from build123d import *

# Parameters (mm, degrees)
SKETCH2_W           = 180
SKETCH2_H           = 300
BOSS_EXTRUDE1_DEPTH = 3
SKETCH3_W           = 8.2
SKETCH3_H           = 260
CUT_EXTRUDE1_DEPTH  = 175.954279742
SKETCH4_R           = 2.5
CUT_EXTRUDE2_DEPTH  = 175.954279742


with BuildPart() as part:
    # Sketch2 → Boss-Extrude1 (new body)
    with BuildSketch(Plane(origin=(0, 0, 0), x_dir=(1, 0, 0), z_dir=(0, 1, 0))):
        Rectangle(SKETCH2_W, SKETCH2_H)
    extrude(amount=BOSS_EXTRUDE1_DEPTH)

    # Sketch3 → Cut-Extrude1 (cut, through all)
    with BuildSketch(Plane(origin=(0, 3, 0), x_dir=(1, 0, 0), z_dir=(0, 1, 0))):
        with Locations((-67.5, 0)):
            Rectangle(SKETCH3_W, SKETCH3_H)
        with Locations((-22.5, 0)):
            Rectangle(SKETCH3_W, SKETCH3_H)
        with Locations((22.5, 0)):
            Rectangle(SKETCH3_W, SKETCH3_H)
        with Locations((67.5, 0)):
            Rectangle(SKETCH3_W, SKETCH3_H)
    extrude(amount=-CUT_EXTRUDE1_DEPTH, mode=Mode.SUBTRACT)

    # Sketch4 → Cut-Extrude2 (cut, through all)
    with BuildSketch(Plane(origin=(0, 3, 0), x_dir=(1, 0, 0), z_dir=(0, 1, 0))):
        with Locations(Location((67.5, -140, 0), (0, 0, 270))):
            Circle(SKETCH4_R)
        with Locations(Location((-67.5, -140, 0), (0, 0, 90))):
            Circle(SKETCH4_R)
        with Locations(Location((67.5, 140, 0), (0, 0, 90))):
            Circle(SKETCH4_R)
        with Locations(Location((-67.5, 140, 0), (0, 0, 270))):
            Circle(SKETCH4_R)
        with Locations(Location((-22.5, -140, 0), (0, 0, 270))):
            Circle(SKETCH4_R)
        with Locations(Location((22.5, -140, 0), (0, 0, 90))):
            Circle(SKETCH4_R)
        with Locations(Location((22.5, 140, 0), (0, 0, 270))):
            Circle(SKETCH4_R)
        with Locations(Location((-22.5, 140, 0), (0, 0, 90))):
            Circle(SKETCH4_R)
    extrude(amount=-CUT_EXTRUDE2_DEPTH, mode=Mode.SUBTRACT)


solid = part.part
Could you check a few things on this model? Use its own coordinates, in mm. Give positions to 0.01 mm unless a question says otherwise; leave off trailing zeros. Order: outer loops, then holes, each group sorted by start corner. A loop starts at its lowest first (then second) coordinate and runs counter-clockwise, first axis right, second up.
1. I need wall thicknesses on L1, parallel to X at y = 1.95, z = 140; L2, parallel to X at y = 1.85, z = -117. Which ranges of each line are inside material? Lowest first, please.
2. Suppose I cut it at A-A (y = 0.75). Give the number of separate pieces and of enclosed holes in the cut face, plus the area to 3 significant figures.
3. Will this pin go through, and if not, where does the flat tip stop? P1, Ø4.5, axis at x = -22.5, z = -140, coming from the -Y side.
4. Suppose I cut it at B-B (z = -23). List the corners of the cut face in (x, y) for me.
Solved:
1. L1: x = -90 to -70, -65 to -25, -20 to 20, 25 to 65, 70 to 90
1. L2: x = -90 to -71.6, -63.4 to -26.6, -18.4 to 18.4, 26.6 to 63.4, 71.6 to 90
2. separate pieces: 1
2. enclosed holes: 12
2. area: 45,300 mm2
3. P1: passes through
4. outline: (-90, 0) - (-71.6, 0) - (-71.6, 3) - (-90, 3) - close; (-63.4, 0) - (-26.6, 0) - (-26.6, 3) - (-63.4, 3) - close; (-18.4, 0) - (18.4, 0) - (18.4, 3) - (-18.4, 3) - close; (26.6, 0) - (63.4, 0) - (63.4, 3) - (26.6, 3) - close; (71.6, 0) - (90, 0) - (90, 3) - (71.6, 3) - close
